from build123d import *

# Parameters (mm, degrees)
ESQUISSE1_W              = 22.8
ESQUISSE1_H              = 12.6
BOSS_EXTRU_1_DEPTH       = 22.5
ESQUISSE2_W              = 31.2
ESQUISSE2_H              = 12.6
BOSS_EXTRU_2_DEPTH       = 2
ENL_V_MAT_EXTRU_1_DEPTH  = 36.0714984
BOSS_EXTRU_3_DEPTH       = 3.99
BOSS_EXTRUDE6_DEPTH      = 1.41
BOSS_EXTRUDE6_DEPTH_BACK = 4
SKETCH1_R                = 4.725
SKETCH1_R_2              = 1.5
SKETCH3_R                = 2.41
BOSS_EXTRUDE7_DEPTH      = 2.78
SKETCH4_R                = 1
CUT_EXTRUDE1_DEPTH       = 9.78
SKETCH8_W                = 1.6
SKETCH8_H                = 1.04
BOSS_EXTRUDE9_DEPTH      = 1.6
CUT_EXTRUDE3_DEPTH       = 43.472296853
MIRROR3_COPY_1_SKETCH_W  = 22.8
MIRROR3_COPY_1_SKETCH_H  = 12.6
MIRROR3_COPY_1_DEPTH     = 22.5
MIRROR3_COPY_2_SKETCH_W  = 1.6
MIRROR3_COPY_2_SKETCH_H  = 1.04
MIRROR3_COPY_2_DEPTH     = 1.6
MIRROR3_COPY_3_DEPTH     = 43.472296853


with BuildPart() as part:
    # Esquisse1 → Boss.-Extru.1 (new body)
    with BuildSketch(Plane.XY):
        with Locations((-11.4, 6.3)):
            Rectangle(ESQUISSE1_W, ESQUISSE1_H)
    boss_extru_1 = extrude(amount=BOSS_EXTRU_1_DEPTH)

    # Esquisse2 → Boss.-Extru.2 (add)
    with BuildSketch(Plane.XY.offset(18.5)):
        with Locations((-11.4, 6.3)):
            Rectangle(ESQUISSE2_W, ESQUISSE2_H)
    extrude(amount=-BOSS_EXTRU_2_DEPTH)

    # Esquisse3 → Enlèv. mat.-Extru.1 (cut, through all)
    with BuildSketch(Plane.XY.offset(18.5)):
        with BuildLine():
            Line((3.745643924, 6.8), (4.2, 6.8))
            Line((4.2, 6.8), (4.2, 5.8))
            Line((4.2, 5.8), (3.745643924, 5.8))
            ThreePointArc((3.745643924, 5.8), (1.35, 6.3), (3.745643924, 6.8))
        make_face()
        with BuildLine():
            Line((-26.545643924, 5.8), (-27, 5.8))
            Line((-27, 5.8), (-27, 6.8))
            Line((-27, 6.8), (-26.545643924, 6.8))
            ThreePointArc((-26.545643924, 6.8), (-24.15, 6.3), (-26.545643924, 5.8))
        make_face()
    extrude(amount=-ENL_V_MAT_EXTRU_1_DEPTH, mode=Mode.SUBTRACT)

    # Esquisse4 → Boss.-Extru.3 (add)
    with BuildSketch(Plane.XY.offset(22.5)):
        with BuildLine():
            Line((-11.15, 9.45), (-11.044039956, 9.45))
            ThreePointArc((-11.044039956, 9.45), (-22.8, 6.3), (-11.044039956, 3.15))
            Line((-11.044039956, 3.15), (-11.15, 3.15))
            ThreePointArc((-11.15, 3.15), (-8, 6.3), (-11.15, 9.45))
        make_face()
    extrude(amount=BOSS_EXTRU_3_DEPTH)

    # Sketch1 → Boss-Extrude6 (add, two sides: drawn at the far end of the back side and taken through both)
    with BuildSketch(Plane.XY.offset(26.49).offset(-BOSS_EXTRUDE6_DEPTH_BACK)):
        with Locations((-16.5, 6.3)):
            Circle(SKETCH1_R)
        with Locations((-10.87, 6.3)):
            Circle(SKETCH1_R_2)
    extrude(amount=BOSS_EXTRUDE6_DEPTH + BOSS_EXTRUDE6_DEPTH_BACK)

    # Sketch3 → Boss-Extrude7 (add)
    with BuildSketch(Plane.XY.offset(27.9)):
        with Locations((-16.5, 6.3)):
            Circle(SKETCH3_R)
    extrude(amount=BOSS_EXTRUDE7_DEPTH)

    # Sketch4 → Cut-Extrude1 (cut)
    with BuildSketch(Plane.XY.offset(30.68)):
        with Locations((-16.5, 6.3)):
            Circle(SKETCH4_R)
    extrude(amount=-CUT_EXTRUDE1_DEPTH, mode=Mode.SUBTRACT)

    # Sketch8 → Boss-Extrude9 (add)
    with BuildSketch(Plane.XY.offset(18.5)):
        with Locations((0.8, 0.52)):
            Rectangle(SKETCH8_W, SKETCH8_H)
    boss_extrude9 = extrude(amount=BOSS_EXTRUDE9_DEPTH)

    # Sketch9 → Cut-Extrude3 (cut, through all)
    with BuildSketch(Plane(origin=(0, 1.04, 0), x_dir=(1, 0, 0), z_dir=(0, 1, 0))):
        Polygon((1.6, -18.5), (0, -20.1), (1.6, -20.1), align=None)
    cut_extrude3 = extrude(amount=-CUT_EXTRUDE3_DEPTH, mode=Mode.SUBTRACT)

    # Mirror1: Boss.-Extru.1, Boss-Extrude9, Cut-Extrude3 across plane
    add(boss_extru_1.mirror(Plane(origin=(0, 6.3, 0), x_dir=(0, 0, 1), z_dir=(0, -1, 0))))
    add(boss_extrude9.mirror(Plane(origin=(0, 6.3, 0), x_dir=(0, 0, 1), z_dir=(0, -1, 0))))
    add(cut_extrude3.mirror(Plane(origin=(0, 6.3, 0), x_dir=(0, 0, 1), z_dir=(0, -1, 0))), mode=Mode.SUBTRACT)

    # Mirror3: Boss.-Extru.1, Boss-Extrude9, Cut-Extrude3 across plane
    add(boss_extru_1.mirror(Plane(origin=(-11.4, 0, 0), x_dir=(0, 0, 1), z_dir=(1, 0, 0))))
    add(boss_extrude9.mirror(Plane(origin=(-11.4, 0, 0), x_dir=(0, 0, 1), z_dir=(1, 0, 0))))
    add(cut_extrude3.mirror(Plane(origin=(-11.4, 0, 0), x_dir=(0, 0, 1), z_dir=(1, 0, 0))), mode=Mode.SUBTRACT)

    # Mirror3 copy 1 sketch → Mirror3 copy 1 (add)
    with BuildSketch(Plane(origin=(-22.8, 12.6, 0), x_dir=(-1, 0, 0), z_dir=(0, 0, 1))):
        with Locations((-11.4, 6.3)):
            Rectangle(MIRROR3_COPY_1_SKETCH_W, MIRROR3_COPY_1_SKETCH_H)
    extrude(amount=MIRROR3_COPY_1_DEPTH)

    # Mirror3 copy 2 sketch → Mirror3 copy 2 (add)
    with BuildSketch(Plane(origin=(-22.8, 12.6, 18.5), x_dir=(-1, 0, 0), z_dir=(0, 0, 1))):
        with Locations((0.8, 0.52)):
            Rectangle(MIRROR3_COPY_2_SKETCH_W, MIRROR3_COPY_2_SKETCH_H)
    extrude(amount=MIRROR3_COPY_2_DEPTH)

    # Mirror3 copy 3 sketch → Mirror3 copy 3 (cut, through all)
    with BuildSketch(Plane(origin=(-22.8, 11.56, 0), x_dir=(-1, 0, 0), z_dir=(0, -1, 0))):
        Polygon((1.6, -18.5), (0, -20.1), (1.6, -20.1), align=None)
    extrude(amount=-MIRROR3_COPY_3_DEPTH, mode=Mode.SUBTRACT)


solid = part.part
Part model, mm, in its own coordinate system. A direction names the side the tool comes from. Coordinates: 2 decimals unless noted, no trailing zeros. Order: outer loops, then holes, each group sorted by start corner. A loop starts at its lowest first (then second) coordinate and runs counter-clockwise, first axis right, second up. Notation, with made-up numbers: M 89.5,80 L 114.5,80 A21 cw 114.5,89 Z; hole C 59,-27 d11. An arc over 180 degrees is marked long. Use a Markdown table: item, result.
(1) Cut at A-A on x = 2.6. Write the cut outline in (y, z), then the cut area to 3 significant figures.
A:
| item | result |
|---|---|
| outline | M 0,16.5 L 5.05,16.5 L 5.05,18.5 L 0,18.5 Z; M 7.55,16.5 L 12.6,16.5 L 12.6,18.5 L 7.55,18.5 Z |
| area | 20.2 mm^2 |
(2) Pull direction Y, two halves, no side cores. Call faces 4 (the cylindrical face through (-22.796, 6.531, 24.467)), 5 (the flat face through (-23, 1.04, 19)), 6 (the flat face through (-22.8, 6, 8)): released by +Y, released by -Y, zero draft, split by the parting line, or undercut.
A:
| item | result |
|---|---|
| face 4 | split by the parting line |
| face 5 | undercut |
| face 6 | zero draft |
(3) Flat gauge pins, fed straight in: pin 1 (3 mm diameter, centred on y = 7.5, z = 22, fed in from +X); pin 2 (3.5 mm diameter, centred on x = -25.4, y = 6.3, fed in from +Z); pin 3 (1.3 mm diameter, centred on x = 3, y = 7, fed in from -Z). Where does each tip first touch, or does it go through?
A:
| item | result |
|---|---|
| pin 1 | stops at x = 0 |
| pin 2 | stops at z = 18.5 |
| pin 3 | stops at z = 16.5 |
(4) Cut at B-B on z = 24. Write the cut outline in (x, y).
A:
| item | result |
|---|---|
| outline | M -11.15,3.15 A3.15 ccw -11.15,9.45 L -11.04,9.45 A6.3 ccw long -11.04,3.15 Z; hole C -16.5,6.3 d2 |
(5) Tool access for faces 1 (the flat face through (-23, 11.56, 19)), 2 (the flat face through (-17, 6, 22.5)), 3 (the flat face through (1, 6, 18.5)): list every direction of +Z, -Z, +X, -X, +Y, -Y with a clear straight run to the whole face (end or side of a thin tool).
A:
| item | result |
|---|---|
| face 1 | +Z, -X |
| face 2 | +Z |
| face 3 | +Z, +X |
(6) Cut at D-D on y = 2. Write the cut outline in (x, z).
A:
| item | result |
|---|---|
| outline | M -27,16.5 L -22.8,16.5 L -22.8,0 L 0,0 L 0,16.5 L 4.2,16.5 L 4.2,18.5 L 0,18.5 L 0,22.5 L -11.9,22.5 L -11.9,26.49 L -14.54,26.49 L -14.54,27.9 L -18.46,27.9 L -18.46,26.49 L -21.1,26.49 L -21.1,22.5 L -22.8,22.5 L -22.8,18.5 L -27,18.5 Z |
(7) Cut at C-C on z = 17.5. Write the cut outline in (x, y).
A:
| item | result |
|---|---|
| outline | M -27,0 L 4.2,0 L 4.2,5.8 L 3.75,5.8 A1.25 cw long 3.75,6.8 L 4.2,6.8 L 4.2,12.6 L -27,12.6 L -27,6.8 L -26.55,6.8 A1.25 cw long -26.55,5.8 L -27,5.8 Z |
(8) Probe L1, parallel to Y at x = -25.4, z = 17.5; L2, parallel to Y at x = -16.5, z = 28; L3, parallel to Z at x = -19.5, y = 2.5. List the from-to ranges inside material, lowest first.
A:
| item | result |
|---|---|
| L1 | y = 0 to 5.05, 7.55 to 12.6 |
| L2 | y = 3.89 to 5.3, 7.3 to 8.71 |
| L3 | z = 0 to 26.49 |
